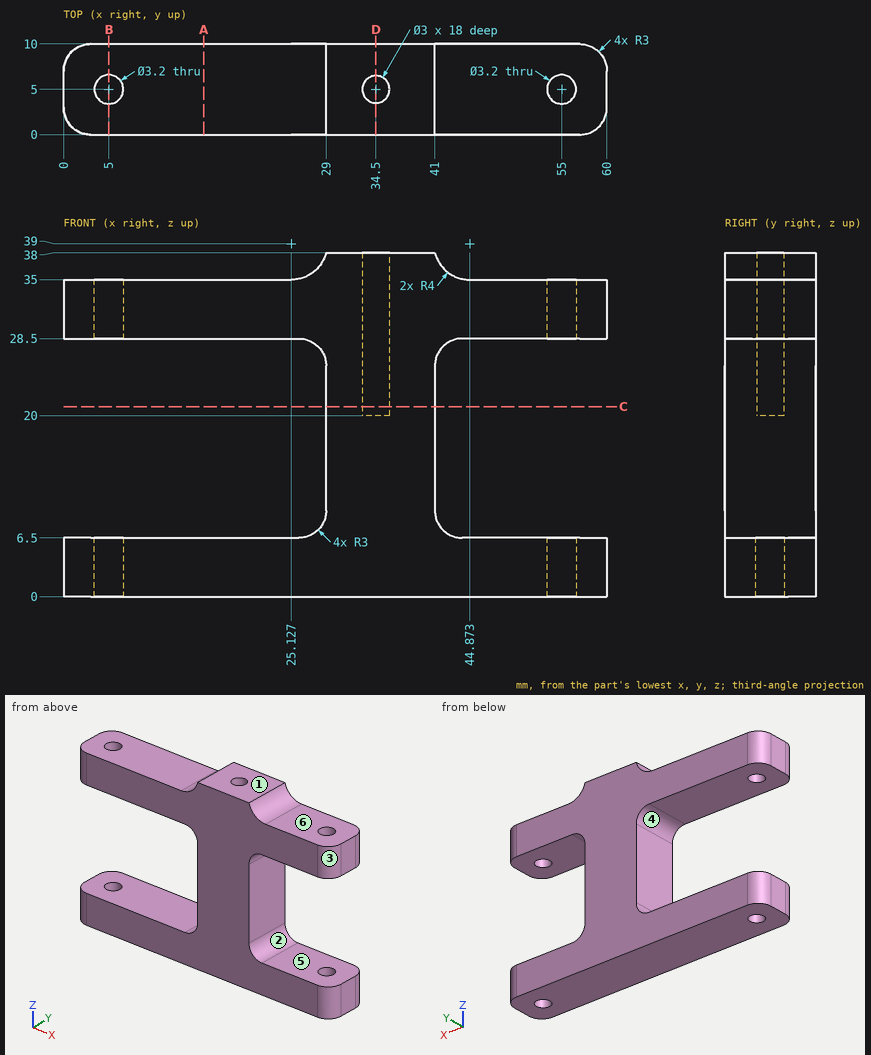
Answer from the drawing. Dimensions are ordinates in mm from the lowest x, y and z of the part. A direction names the side the tool comes from. Round coordinates to 2 decimals unless told otherwise and drop trailing zeros. Order: outer loops, then holes, each group sorted by start corner. A loop starts at its lowest first (then second) coordinate and runs counter-clockwise, first axis right, second up.
1) For the marked faces 4, 5 and 6, determine the directions among +Z, -Z, +X, -X, +Y, -Y from which every point of the face is accessible in a straight line to the end or side of a thin tool.
2) The part is cut by section C-C on z = 21. Write down the section's boundary in (x, y).
3) Flat-ended cylindrical pins translate along their axes: pin 1 (1.5 mm diameter, centred on y = 1, z = 9.5, fed in from -X); pin 2 (5 mm diameter, centred on x = 5, y = 5, fed in from +Z); pin 3 (2.5 mm diameter, centred on x = 5, y = 5, fed in from -Z); pin 4 (3 mm diameter, centred on y = 4.5, z = 17.5, fed in from +X). Find the tip coordinate at first contact, or state that the pin passes through.
4) The mould has two halves that part along Z. Classify the marked faces 1, 2 and 3: released by +Z, released by -Z, zero draft, split by the parting line, or undercut.
5) The part is cut by section A-A on x = 15.5. Write down the section's boundary in (y, z), plus the area to 3 significant figures.
6) The part is cut by section B-B on x = 5. Write down the section's boundary in (y, z), plus the area to 3 significant figures.
7) Straight lines are drawn through the part: L1, parallel to Z at x = 51, y = 4.25; L2, parallel to Y at x = 5, z = 1.5; L3, parallel to X at y = 9, z = 13.5. For each, find the intervals that lie inside material, in ascending order.
8) The part is cut by section D-D on x = 34.5. Write down the section's boundary in (y, z), plus the area to 3 significant figures.
Resolved:
1. face 4: -X, +Y, -Y
1. face 5: +X, +Y, -Y
1. face 6: +Z, +X, +Y, -Y
2. outline: (29, 0) - (41, 0) - (41, 10) - (29, 10) - close; hole circle Ø3 at (34.5, 5)
3. pin 1: stops at x = 28.9
3. pin 2: stops at z = 35
3. pin 3: passes through
3. pin 4: stops at x = 41
4. face 1: released by +Z
4. face 2: undercut
4. face 3: zero draft
5. outline: (0, 0) - (10, 0) - (10, 6.5) - (0, 6.5) - close; (0, 28.5) - (10, 28.5) - (10, 35) - (0, 35) - close
5. area: 130 mm2
6. outline: (0, 0) - (3.4, 0) - (3.4, 6.5) - (0, 6.5) - close; (0, 28.5) - (3.4, 28.5) - (3.4, 35) - (0, 35) - close; (6.6, 0) - (10, 0) - (10, 6.5) - (6.6, 6.5) - close; (6.6, 28.5) - (10, 28.5) - (10, 35) - (6.6, 35) - close
6. area: 88.4 mm2
7. L1: z = 0 to 6.5, 28.5 to 35
7. L2: y = 0 to 3.4, 6.6 to 10
7. L3: x = 29 to 41
8. outline: (0, 0) - (10, 0) - (10, 38) - (6.5, 38) - (6.5, 20) - (3.5, 20) - (3.5, 38) - (0, 38) - close
8. area: 326 mm2
